Check sheet for the modelled part. Datum: model origin and axes. Units: mm. A direction names the side the tool comes from. Round coordinates to 2 decimals unless told otherwise and drop trailing zeros. Write each loop counter-clockwise with the first axis right and the second up, starting at its lowest first coordinate (ties: lowest second). Pieces come first, ordered by that corner, then holes.
from build123d import *

# Parameters (mm, degrees)
SKETCH_1_R           = 11
EXTRUDE_1_DEPTH      = 50
SKETCH_2_W           = 6
SKETCH_2_H           = 6
EXTRUDE_2_DEPTH      = 0.1
EXTRUDE_2_DEPTH_BACK = 25
CHAMFER_1_SIZE       = 1
SKETCH_3_R           = 100
EXTRUDE_3_DEPTH      = 10
SKETCH_4_R           = 65
SKETCH_4_R_2         = 60
EXTRUDE_4_DEPTH      = 3.5
SKETCH_5_R           = 60
SKETCH_5_R_2         = 18
CUT_EXTRUDE_1_DEPTH  = 3.5
CHAMFER_2_SIZE       = 1
SKETCH_6_R           = 65
EXTRUDE_5_DEPTH      = 30
SKETCH_7_R           = 71
EXTRUDE_6_DEPTH      = 149
SKETCH_8_R           = 72.248091185
EXTRUDE_7_DEPTH      = 81.5
CHAMFER_3_SIZE       = 26
SKETCH_9_R           = 6
CUT_EXTRUDE_2_DEPTH  = 271.5
EXTRUDE_8_DEPTH      = 124
CUT_EXTRUDE_3_REACH  = 182
SKETCH_11_R          = 5
SKETCH_12_W          = 60
SKETCH_12_H          = 60
EXTRUDE_9_DEPTH      = 124.5
SKETCH_13_R          = 15
EXTRUDE_10_DEPTH     = 76.5
CHAMFER_4_SIZE       = 1
SKETCH_15_R          = 6
SKETCH_16_R          = 8
EXTRUDE_11_DEPTH     = 6
EXTRUDE_12_DEPTH     = 10
SKETCH_18_R          = 6
CUT_EXTRUDE_4_DEPTH  = 10


with BuildPart() as part:
    # Эскиз1 → Вытянуть1 (new body)
    with BuildSketch(Plane.XY):
        Circle(SKETCH_1_R)
    extrude(amount=EXTRUDE_1_DEPTH)

    # Эскиз2 → Вытянуть2 (add, two sides)
    with BuildSketch(Plane(origin=(0, 0, 0), x_dir=(-1, 0, 0), z_dir=(0, 0, -1))) as extrude_2_sk:
        with Locations((0, 10.5)):
            Rectangle(SKETCH_2_W, SKETCH_2_H)
    extrude(amount=EXTRUDE_2_DEPTH)
    extrude(extrude_2_sk.sketch, amount=-EXTRUDE_2_DEPTH_BACK)

    # Фаска1
    chamfer_1_edges = [part.edges().sort_by_distance(p)[0] for p in [
        (-6.633249581, -8.774964387, 0),
    ]]
    chamfer(chamfer_1_edges, length=CHAMFER_1_SIZE)

    # Эскиз3 → Вытянуть3 (add)
    with BuildSketch(Plane.XY.offset(50)):
        Circle(SKETCH_3_R)
    extrude(amount=EXTRUDE_3_DEPTH)

    # Эскиз4 → Вытянуть4 (add)
    with BuildSketch(Plane(origin=(0, 0, 50), x_dir=(-1, 0, 0), z_dir=(0, 0, -1))):
        with Locations(Location((0, 0, 0), (0, 0, 180))):  # turned: the seam where the file's is
            Circle(SKETCH_4_R)
        Circle(SKETCH_4_R_2, mode=Mode.SUBTRACT)
    extrude(amount=EXTRUDE_4_DEPTH)

    # Эскиз5 → Вырез-Вытянуть1 (cut)
    with BuildSketch(Plane(origin=(0, 0, 50), x_dir=(-1, 0, 0), z_dir=(0, 0, -1))):
        Circle(SKETCH_5_R)
        Circle(SKETCH_5_R_2, mode=Mode.SUBTRACT)
    extrude(amount=-CUT_EXTRUDE_1_DEPTH, mode=Mode.SUBTRACT)

    # Фаска2
    chamfer_2_edges = [part.edges().sort_by_distance(p)[0] for p in [
        (-65, 0, 46.5),
        (18, 0, 50),
    ]]
    chamfer(chamfer_2_edges, length=CHAMFER_2_SIZE)

    # Эскиз6 → Вытянуть5 (add)
    with BuildSketch(Plane.XY.offset(60)):
        Circle(SKETCH_6_R)
    extrude(amount=EXTRUDE_5_DEPTH)

    # Эскиз7 → Вытянуть6 (add)
    with BuildSketch(Plane.XY.offset(90)):
        Circle(SKETCH_7_R)
    extrude(amount=EXTRUDE_6_DEPTH)

    # Эскиз8 → Вытянуть7 (add)
    with BuildSketch(Plane.XY.offset(239)):
        Circle(SKETCH_8_R)
    extrude(amount=EXTRUDE_7_DEPTH)

    # Фаска3
    chamfer_3_edges = [part.edges().sort_by_distance(p)[0] for p in [
        (-72.248091185, 0, 320.5),
    ]]
    chamfer(chamfer_3_edges, length=CHAMFER_3_SIZE)

    # Эскиз9 → Вырез-Вытянуть2 (cut, through all)
    with BuildSketch(Plane(origin=(0, 0, 50), x_dir=(-1, 0, 0), z_dir=(0, 0, -1))):
        with Locations((-31.57138317, 76.220061432)):
            Circle(SKETCH_9_R)
        with Locations((31.57138317, 76.220061432)):
            Circle(SKETCH_9_R)
        with Locations((76.220061432, 31.57138317)):
            Circle(SKETCH_9_R)
        with Locations((76.220061432, -31.57138317)):
            Circle(SKETCH_9_R)
        with Locations((31.57138317, -76.220061432)):
            Circle(SKETCH_9_R)
        with Locations((-31.57138317, -76.220061432)):
            Circle(SKETCH_9_R)
        with Locations((-76.220061432, -31.57138317)):
            Circle(SKETCH_9_R)
        with Locations((-76.220061432, 31.57138317)):
            Circle(SKETCH_9_R)
    extrude(amount=-CUT_EXTRUDE_2_DEPTH, mode=Mode.SUBTRACT)

    # Эскиз10 → Вытянуть8 (add)
    with BuildSketch(Plane(origin=(0, 0, 90), x_dir=(-1, 0, 0), z_dir=(0, 0, -1))):
        Polygon((-74.5, -80), (-48.088457268, -80), (-11.515477308, -58.884580175), (-23.295059446, -55.293220248), (-50.5, -71), (-74.5, -71), align=None)
        Polygon((74.5, -71), (74.5, -80), (48.088457268, -80), (11.515477308, -58.884580175), (23.295059446, -55.293220248), (50.5, -71), align=None)
    extrude(amount=-EXTRUDE_8_DEPTH)

    # Эскиз11 → Вырез-Вытянуть3 (cut, up to next)
    with BuildSketch(Plane.XZ.offset(80), mode=Mode.PRIVATE) as cut_extrude_3_sk1:
        with Locations(Location((-62.5, 100, 0), (0, 0, 270))):  # turned: the seam where the file's is
            Circle(SKETCH_11_R)
    cut_extrude_3_tool1 = extrude(cut_extrude_3_sk1.sketch, amount=-CUT_EXTRUDE_3_REACH, mode=Mode.PRIVATE) & part.part
    add(cut_extrude_3_tool1.solids().sort_by_distance((-62.5, -80, 100))[0], mode=Mode.SUBTRACT)
    # Эскиз11 → Вырез-Вытянуть3 (cut, up to next)
    with BuildSketch(Plane.XZ.offset(80), mode=Mode.PRIVATE) as cut_extrude_3_sk2:
        with Locations(Location((62.5, 100, 0), (0, 0, 270))):  # turned: the seam where the file's is
            Circle(SKETCH_11_R)
    cut_extrude_3_tool2 = extrude(cut_extrude_3_sk2.sketch, amount=-CUT_EXTRUDE_3_REACH, mode=Mode.PRIVATE) & part.part
    add(cut_extrude_3_tool2.solids().sort_by_distance((62.5, -80, 100))[0], mode=Mode.SUBTRACT)
    # Эскиз11 → Вырез-Вытянуть3 (cut, up to next)
    with BuildSketch(Plane.XZ.offset(80), mode=Mode.PRIVATE) as cut_extrude_3_sk3:
        with Locations(Location((-62.5, 200, 0), (0, 0, 270))):  # turned: the seam where the file's is
            Circle(SKETCH_11_R)
    cut_extrude_3_tool3 = extrude(cut_extrude_3_sk3.sketch, amount=-CUT_EXTRUDE_3_REACH, mode=Mode.PRIVATE) & part.part
    add(cut_extrude_3_tool3.solids().sort_by_distance((-62.5, -80, 200))[0], mode=Mode.SUBTRACT)
    # Эскиз11 → Вырез-Вытянуть3 (cut, up to next)
    with BuildSketch(Plane.XZ.offset(80), mode=Mode.PRIVATE) as cut_extrude_3_sk4:
        with Locations(Location((62.5, 200, 0), (0, 0, 270))):  # turned: the seam where the file's is
            Circle(SKETCH_11_R)
    cut_extrude_3_tool4 = extrude(cut_extrude_3_sk4.sketch, amount=-CUT_EXTRUDE_3_REACH, mode=Mode.PRIVATE) & part.part
    add(cut_extrude_3_tool4.solids().sort_by_distance((62.5, -80, 200))[0], mode=Mode.SUBTRACT)

    # Эскиз12 → Вытянуть9 (add)
    with BuildSketch(Plane(origin=(0, 0, 0), x_dir=(1, 0, 0), z_dir=(0, 1, 0))):
        with Locations((0, -121)):
            Rectangle(SKETCH_12_W, SKETCH_12_H)
    extrude(amount=EXTRUDE_9_DEPTH)

    # Эскиз13 → Вытянуть10 (add)
    with BuildSketch(Plane(origin=(0, 0, 0), x_dir=(1, 0, 0), z_dir=(0, 1, 0))):
        with Locations(Location((0, -175, 0), (0, 0, 90))):  # turned: the seam where the file's is
            Circle(SKETCH_13_R)
    extrude(amount=EXTRUDE_10_DEPTH)

    # Фаска4
    chamfer_4_edges = [part.edges().sort_by_distance(p)[0] for p in [
        (0, 76.5, 190),
    ]]
    chamfer(chamfer_4_edges, length=CHAMFER_4_SIZE)

    # По траектории1: sweep along a path in Эскиз14
    with BuildLine(Plane.XY.offset(175)) as sweep_1_path:
        CenterArc((0, 91.5), 15, 0, 360)
    # Эскиз15 → По траектории1 (sweep)
    with BuildSketch(Plane(origin=(0, 0, 0), x_dir=(0, 0, -1), z_dir=(1, 0, 0))):
        with Locations((-175, 106.5)):
            Circle(SKETCH_15_R)
    sweep(path=sweep_1_path.line)

    # Эскиз16 → Вытянуть11 (add)
    with BuildSketch(Plane.ZY.offset(30)):
        with Locations(Location((121, 94.5, 0), (0, 0, 180))):  # turned: the seam where the file's is
            Circle(SKETCH_16_R)
    extrude(amount=EXTRUDE_11_DEPTH)

    # Эскиз17 → Вытянуть12 (add)
    with BuildSketch(Plane.ZY.offset(36)):
        Polygon((121, 110.088457268), (107.5, 102.294228634), (107.5, 86.705771366), (121, 78.911542732), (134.5, 86.705771366), (134.5, 102.294228634), align=None)
    extrude(amount=EXTRUDE_12_DEPTH)

    # Эскиз18 → Вырез-Вытянуть4 (cut)
    with BuildSketch(Plane.ZY.offset(46)):
        with Locations((121, 94.5)):
            Circle(SKETCH_18_R)
    extrude(amount=-CUT_EXTRUDE_4_DEPTH, mode=Mode.SUBTRACT)


solid = part.part
1. Sectioned sample at B-B, the plane z = 139. Enter the section's corners in (x, y), plus the area to 3 significant figures.
2. Set-up check for faces 1 (the flat face through (74.5, -75, 151)), 2 (the cylindrical face through (62, -19.52, 48.77)), 3 (the cylindrical face through (68.912, 21.701, 266.362)), 4 (the flat face through (-46, 94.7, 114.8)), 5 (the flat face through (0, -66, 90)): record each of +Z, -Z, +X, -X, +Y, -Y from which the full face is reachable in a straight line by a thin tool's end or side.
3. Release check for a two-part mould opening along Y. For faces 6 (the cylindrical face through (66.716, -75.563, 97.312)), 7 (the cylindrical face through (32.872, -82.077, 54.93)), 8 (the flat face through (0, 124.5, 121)) record: released by +Y, released by -Y, zero draft, split by the parting line, or undercut.
4. Sectioned sample at C-C, the plane z = 82. Enter the section's corners in (x, y), plus the area to 3 significant figures.
5. Go/stop test with flat-tipped pins: pin 1 (1.5 mm diameter, centred on y = -54, z = 83, fed in from +X); pin 2 (10 mm diameter, centred on x = -79.5, z = 49.5, fed in from +Y); pin 3 (1.5 mm diameter, centred on y = -8.5, z = 34, fed in from +X). Record where each tip stops, or that it passes through.
6. Sectioned sample at A-A, the plane z = 200. Enter the section's corners in (x, y).
7. Scan lines: line 1 along Y through (x, z) = (0, 49); line 2 along Z through (x, y) = (-62, -75); line 3 along X through (y, z) = (91, 113). Record each from-to range of solid material in increasing order.
Computed values:
1. outline: (-74.5, -80) - (-48.09, -80) - (-24.77, -66.54) arc R71 ccw to (24.77, -66.54) - (48.09, -80) - (74.5, -80) - (74.5, -71) - (50.5, -71) - (34.76, -61.91) arc R71 ccw to (30, 64.35) - (30, 124.5) - (-30, 124.5) - (-30, 64.35) arc R71 ccw to (-34.76, -61.91) - (-50.5, -71) - (-74.5, -71) - close
1. area: 20,000 mm2
2. face 1: +Z, -Z, +X, +Y, -Y
2. face 2: -Z
2. face 3: +Z
2. face 4: +Z, -X, +Y
2. face 5: none
3. face 6: zero draft
3. face 7: undercut
3. face 8: released by +Y
4. outline: circle Ø130 at (0, 0)
4. area: 13,300 mm2
5. pin 1: stops at x = 37.28
5. pin 2: stops at y = 66.68
5. pin 3: stops at x = 7.81
6. outline: (-74.5, -80) - (-67.5, -80) - (-67.5, -71) - (-74.5, -71) - close; (-57.5, -80) - (-48.09, -80) - (-24.77, -66.54) arc R71 ccw to (24.77, -66.54) - (48.09, -80) - (57.5, -80) - (57.5, -71) - (50.5, -71) - (34.76, -61.91) arc R71 ccw (long way) to (-34.76, -61.91) - (-50.5, -71) - (-57.5, -71) - close; (67.5, -80) - (74.5, -80) - (74.5, -71) - (67.5, -71) - close
7. line 1: y = -65 to -60, -11 to 11, 60 to 65
7. line 2: z = 50 to 60, 90 to 95.03, 104.97 to 195.03, 204.97 to 214
7. line 3: x = -46 to -36, -30 to 30
